Could you check a few things on this model? Use its own coordinates, in mm. Give positions to 0.01 mm unless a question says otherwise; leave off trailing zeros. Loops run counter-clockwise (first coordinate to the right, second up) from the corner with the lowest first, then second, coordinate; pieces in that order, holes last. Notation, with made-up numbers: M -37,28.25 L -3,28.25 A18 cw -3,45.25 Z; hole C 46.5,-19.5 d6. An arc over 180 degrees is marked long. Use CSV: the item, a comma, the result in double quotes.
```python
from build123d import *

# Parameters (mm, degrees)
SKETCH1_W           = 228.6
SKETCH1_H           = 31.75
BOSS_EXTRUDE1_DEPTH = 3.175
SKETCH2_R           = 2.032
CUT_EXTRUDE1_DEPTH  = 3.175
SKETCH3_W           = 76.2
SKETCH3_H           = 15.494
CUT_EXTRUDE2_DEPTH  = 3.175


with BuildPart() as part:
    # Sketch1 → Boss-Extrude1 (new body)
    with BuildSketch(Plane(origin=(0, 0, 0), x_dir=(1, 0, 0), z_dir=(0, 1, 0))):
        with Locations((114.3, 15.875)):
            Rectangle(SKETCH1_W, SKETCH1_H)
    extrude(amount=BOSS_EXTRUDE1_DEPTH)

    # Sketch2 → Cut-Extrude1 (cut)
    with BuildSketch(Plane(origin=(0, 3.175, 0), x_dir=(1, 0, 0), z_dir=(0, 1, 0))):
        with Locations((5.08, 19.05)):
            Circle(SKETCH2_R)
        with Locations((223.52, 19.05)):
            Circle(SKETCH2_R)
    extrude(amount=-CUT_EXTRUDE1_DEPTH, mode=Mode.SUBTRACT)

    # Sketch3 → Cut-Extrude2 (cut)
    with BuildSketch(Plane(origin=(0, 3.175, 0), x_dir=(1, 0, 0), z_dir=(0, 1, 0))):
        with Locations((119.38, 17.907)):
            Rectangle(SKETCH3_W, SKETCH3_H)
    extrude(amount=-CUT_EXTRUDE2_DEPTH, mode=Mode.SUBTRACT)


solid = part.part
```
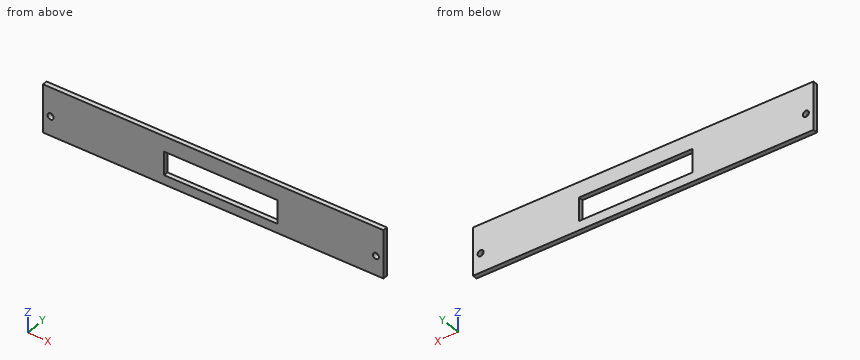
1. I want a section at A-A, the plane z = -19.05. List the corners of the cut face in (x, y) for me (3 decimals), then the cut area to 3 significant figures.
Outcome:
outline,"M 0,0 L 3.048,0 L 3.048,3.175 L 0,3.175 Z; M 7.112,0 L 81.28,0 L 81.28,3.175 L 7.112,3.175 Z; M 157.48,0 L 221.488,0 L 221.488,3.175 L 157.48,3.175 Z; M 225.552,0 L 228.6,0 L 228.6,3.175 L 225.552,3.175 Z"
area,"458 mm2"
2. I want a section at B-B, the plane x = 96.5. List the corners of the cut face in (y, z) for me (3 decimals), then the cut area to 3 significant figures.
Outcome:
outline,"M 0,-31.75 L 3.175,-31.75 L 3.175,-25.654 L 0,-25.654 Z; M 0,-10.16 L 3.175,-10.16 L 3.175,0 L 0,0 Z"
area,"51.6 mm2"
3. I want a section at D-D, the plane x = 5.08. List the corners of the cut face in (y, z) for me (3 decimals), then the cut area to 3 significant figures.
Outcome:
outline,"M 0,-31.75 L 3.175,-31.75 L 3.175,-21.082 L 0,-21.082 Z; M 0,-17.018 L 3.175,-17.018 L 3.175,0 L 0,0 Z"
area,"87.9 mm2"
4. Please list where these lines run through material, in increasing order: line 1 (X direction, y = 2, z = -19.05); line 2 (Z direction, x = 223.52, y = 1.9); line 3 (X direction, y = 1.6, z = -12.5).
Outcome:
line 1,"0 to 3.05, 7.11 to 81.28, 157.48 to 221.49, 225.55 to 228.6"
line 2,"-31.75 to -21.08, -17.02 to 0"
line 3,"0 to 81.28, 157.48 to 228.6"
5. I want a section at C-C, the plane y = 0.5. List the corners of the cut face in (x, z) for me, then the cut area to 3 significant figures.
Outcome:
outline,"M 0,-31.75 L 228.6,-31.75 L 228.6,0 L 0,0 Z; hole C 5.08,-19.05 d4.06; hole M 81.28,-25.65 L 157.48,-25.65 L 157.48,-10.16 L 81.28,-10.16 Z; hole C 223.52,-19.05 d4.06"
area,"6,050 mm2"
